```python
from build123d import *

# Parameters (mm, degrees)
SKETCH2_W                  = 100
SKETCH2_H                  = 100
BOSS_EXTRUDE1_DEPTH        = 12
SKETCH3_R                  = 16
CUT_EXTRUDE1_DEPTH         = 10
M6_CLEARANCE_HOLE1_D       = 6.1
BOSS_EXTRUDE2_START        = 30
SKETCH17_R                 = 3.05
BOSS_EXTRUDE2_DEPTH        = 30
CIRPATTERN1_COUNT          = 4
SKETCH18_R                 = 14
CUT_EXTRUDE3_DEPTH         = 77.811457479
FILLET1_R                  = 2
FILLET2_R                  = 7
CUT_EXTRUDE6_DEPTH         = 5
CIRPATTERN2_COUNT          = 4
SKETCH25_R                 = 30
SKETCH25_R_2               = 14
BOSS_EXTRUDE3_DEPTH        = 2
F_8_0_199_DIAMETER_HOLE1_D = 5.0546
CHAMFER1_SIZE              = 0.5
FILLET3_R                  = 1


with BuildPart() as part:
    # Sketch2 → Boss-Extrude1 (new body)
    with BuildSketch(Plane.XY):
        Rectangle(SKETCH2_W, SKETCH2_H)
    extrude(amount=BOSS_EXTRUDE1_DEPTH)

    # Sketch3 → Cut-Extrude1 (cut)
    with BuildSketch(Plane(origin=(0, 0, 0), x_dir=(-1, 0, 0), z_dir=(0, 0, -1))):
        Circle(SKETCH3_R)
    extrude(amount=-CUT_EXTRUDE1_DEPTH, mode=Mode.SUBTRACT)

    # M6 Clearance Hole1 (through all)
    with Locations(Plane(origin=(0, 0, 12), x_dir=(-1, 0, 0), z_dir=(0, 0, 1))):
        with Locations((42.5, -42.5), (-42.5, 42.5), (-42.5, -42.5), (42.5, 42.5)):
            Hole(M6_CLEARANCE_HOLE1_D / 2)

    # Sketch17 → Boss-Extrude2 (add)
    with BuildSketch(Plane(origin=(0, 0, 0), x_dir=(-1, 0, 0), z_dir=(0, 0, -1)).offset(BOSS_EXTRUDE2_START)):
        with BuildLine():
            Line((-37.45, 42.5), (-37.45, 50))
            Line((-37.45, 50), (-50, 50))
            Line((-50, 50), (-50, 37.45))
            Line((-50, 37.45), (-42.5, 37.45))
            ThreePointArc((-42.5, 37.45), (-38.929110755, 38.929110755), (-37.45, 42.5))
        make_face()
        with Locations(Location((-42.5, 42.5, 0), (0, 0, 180))):
            Circle(SKETCH17_R, mode=Mode.SUBTRACT)
    boss_extrude2 = extrude(amount=-BOSS_EXTRUDE2_DEPTH)

    # CirPattern1: Boss-Extrude2 ×4 about axis
    cirpattern1_axis = Axis((0, 0, 0), (0, 0, 1))
    for i in range(1, CIRPATTERN1_COUNT):
        add(boss_extrude2.rotate(cirpattern1_axis, i * 360 / CIRPATTERN1_COUNT))

    # Sketch18 → Cut-Extrude3 (cut, through all)
    with BuildSketch(Plane(origin=(0, 0, 0), x_dir=(-1, 0, 0), z_dir=(0, 0, -1))):
        Circle(SKETCH18_R)
    extrude(amount=-CUT_EXTRUDE3_DEPTH, mode=Mode.SUBTRACT)

    # Fillet1
    fillet1_edges = [part.edges().sort_by_distance(p)[0] for p in [
        (38.929110755, 38.929110755, 0),
        (37.45, 46.25, 0),
        (46.25, 37.45, 0),
        (-38.929110755, 38.929110755, 0),
        (-46.25, 37.45, 0),
        (-37.45, 46.25, 0),
        (-38.929110755, -38.929110755, 0),
        (-37.45, -46.25, 0),
        (-46.25, -37.45, 0),
        (38.929110755, -38.929110755, 0),
        (46.25, -37.45, 0),
        (37.45, -46.25, 0),
    ]]
    fillet(fillet1_edges, radius=FILLET1_R)

    # Fillet2
    fillet2_edges = [part.edges().sort_by_distance(p)[0] for p in [
        (50, -50, -9),
        (-50, -50, -9),
        (-50, 50, -9),
        (50, 50, -9),
    ]]
    fillet(fillet2_edges, radius=FILLET2_R)

    # Sketch24 → Cut-Extrude6 (cut)
    with BuildSketch(Plane.XY.offset(12)):
        Polygon((-44.400625379, 48.073833795), (-48.277394352, 43.640927036), (-46.376768973, 38.067093242), (-40.599374621, 36.926166205), (-36.722605648, 41.359072964), (-38.623231027, 46.932906758), align=None)
    cut_extrude6 = extrude(amount=-CUT_EXTRUDE6_DEPTH, mode=Mode.SUBTRACT)

    # CirPattern2: Cut-Extrude6 ×4 about axis
    cirpattern2_axis = Axis((0, 0, 0), (0, 0, 1))
    for i in range(1, CIRPATTERN2_COUNT):
        add(cut_extrude6.rotate(cirpattern2_axis, i * 360 / CIRPATTERN2_COUNT), mode=Mode.SUBTRACT)

    # Sketch25 → Boss-Extrude3 (add)
    with BuildSketch(Plane.XY.offset(12)):
        with Locations(Location((0, 0, 0), (0, 0, 180))):
            Circle(SKETCH25_R)
        with Locations(Location((0, 0, 0), (0, 0, 180))):
            Circle(SKETCH25_R_2, mode=Mode.SUBTRACT)
    extrude(amount=BOSS_EXTRUDE3_DEPTH)

    # #8 (0.199) Diameter Hole1 (through all)
    with Locations(Plane(origin=(26.516504294, 26.516504294, 12), x_dir=(1, 0, 0), z_dir=(0, 0, 1))):
        with Locations((0, 0), (-53.033008588, 0), (-53.033008588, -53.033008588), (0, -53.033008588)):
            Hole(F_8_0_199_DIAMETER_HOLE1_D / 2)

    # Chamfer1
    chamfer1_edges = [part.edges().sort_by_distance(p)[0] for p in [
        (30, 0, 14),
    ]]
    chamfer(chamfer1_edges, length=CHAMFER1_SIZE)

    # Fillet3
    fillet3_edges = [part.edges().sort_by_distance(p)[0] for p in [
        (50, 0, 0),
        (0, -50, 0),
        (-50, 0, 0),
        (0, 50, 0),
        (-36.864213562, 50, -0.585786438),
        (-50, 36.864213562, -0.585786438),
        (-50, -36.864213562, -0.585786438),
        (-36.864213562, -50, -0.585786438),
        (36.864213562, -50, -0.585786438),
        (50, -36.864213562, -0.585786438),
        (50, 36.864213562, -0.585786438),
        (36.864213562, 50, -0.585786438),
        (37.45, 50, -16),
        (50, 37.45, -16),
        (-50, 37.45, -16),
        (-37.45, 50, -16),
        (-37.45, -50, -16),
        (-50, -37.45, -16),
        (50, -37.45, -16),
        (37.45, -50, -16),
    ]]
    fillet(fillet3_edges, radius=FILLET3_R)


solid = part.part
```
Geometry: final body of the model. Coordinates: model frame, mm. A direction names the side the tool comes from. Give positions to 0.01 mm unless a question says otherwise; leave off trailing zeros. Order: outer loops, then holes, each group sorted by start corner. A loop starts at its lowest first (then second) coordinate and runs counter-clockwise, first axis right, second up. Notation, with made-up numbers: M -25,36.25 L -17,36.25 A16 cw -17,50.25 Z; hole C 57,73.25 d1. An arc over 180 degrees is marked long. Answer as CSV lines item,"result". Start each with the question number.
1) Line query: line 1 (Y direction, x = 42.5, z = -6); line 2 (X direction, y = 0, z = 11); line 3 (Y direction, x = 0, z = 7). Output: solid intervals per line, ascending. Write a range as from..to.
2) First-contact query: P1, Ø2, axis at x = -26.5, y = -15.5, coming from the +Z side; P2, Ø5.5, axis at x = 44, y = 45.5, coming from the +Z side; P3, Ø6, axis at y = 35, z = -18, coming from the +X side. Flat tips, straight axial feed; report the tip coordinate or a pass-through.
3) Set-up query: faces 1 (the flat face through (0, -50, 2)), 2 (the flat face through (-46, -37.45, -16)), 3 (the cylindrical face through (38.89, -38.97, -16.2)), 4 (the flat face through (-37.5, -43.5, 9.5)). Return all of +Z, -Z, +X, -X, +Y, -Y with unobstructed straight access to the full face (end or side cutting, diameter ignored); none if empty.
4) Mould query, pull axis X, two halves, no side actions, for faces 5 (the flat face through (45, 45, -30)), 6 (the cylindrical face through (48, 47.9, -9.3)), 7 (the flat face through (-12, 12, 0)), 8 (the flat face through (37.66, -44.11, 9.54)). Classes: +X half, -X half, draft (parallel to the pull), parting line (faces both ways), or undercut.
5) Cut plane A-A (x = 0). Output: boundary loops of the cut face in (y, z), then the cut area to 3 significant figures.
6) Cut plane B-B (z = -18). State how many separate pieces and enclosed holes the cut face has, then the cut area to 3 significant figures.
Findings below:
1,line 1,"y = -50..-45.55, -39.45..-37.45, 37.45..39.45, 45.55..50"
1,line 2,"x = -50..-14, 14..50"
1,line 3,"y = -50..-16, 16..50"
2,P1,"stops at z = 13.8"
2,P2,"stops at z = 12"
2,P3,"stops at x = 49.89"
3,face 1,"+Z, -Z, +X, -X, -Y"
3,face 2,"-Z, +X, -X"
3,face 3,"-Z"
3,face 4,"+Z"
4,face 5,"draft"
4,face 6,"+X half"
4,face 7,"undercut"
4,face 8,"undercut"
5,outline,"M -50,1 A1 ccw -49,0 L -16,0 L -16,10 L -14,10 L -14,14 L -29.5,14 L -30,13.5 L -30,12 L -50,12 Z; M 14,10 L 16,10 L 16,0 L 49,0 A1 ccw 50,1 L 50,12 L 30,12 L 30,13.5 L 29.5,14 L 14,14 Z"
5,area,"887 mm²"
6,separate pieces,"4"
6,enclosed holes,"4"
6,area,"447 mm²"
